from build123d import *

# Parameters (mm, degrees)
SKETCH1_R               = 30
SKETCH1_R_2             = 2
SKETCH1_R_3             = 6
BOSS_EXTRUDE1_DEPTH     = 12
SKETCH2_R               = 2.5
CUT_EXTRUDE1_DEPTH      = 31
CUT_EXTRUDE1_DEPTH_BACK = 31
SKETCH3_R               = 5
CUT_EXTRUDE2_DEPTH      = 5


with BuildPart() as part:
    # Sketch1 → Boss-Extrude1 (new body)
    with BuildSketch(Plane(origin=(0, 0, 0), x_dir=(1, 0, 0), z_dir=(0, 1, 0))):
        Circle(SKETCH1_R)
        with Locations((20, 0)):
            Circle(SKETCH1_R_2, mode=Mode.SUBTRACT)
        with Locations((10, -17.320508076)):
            Circle(SKETCH1_R_2, mode=Mode.SUBTRACT)
        with Locations((-10, -17.320508076)):
            Circle(SKETCH1_R_2, mode=Mode.SUBTRACT)
        with Locations((-20, 0)):
            Circle(SKETCH1_R_2, mode=Mode.SUBTRACT)
        with Locations((-10, 17.320508076)):
            Circle(SKETCH1_R_2, mode=Mode.SUBTRACT)
        with Locations((10, 17.320508076)):
            Circle(SKETCH1_R_2, mode=Mode.SUBTRACT)
        Circle(SKETCH1_R_3, mode=Mode.SUBTRACT)
    extrude(amount=BOSS_EXTRUDE1_DEPTH)

    # Sketch2 → Cut-Extrude1 (cut, two sides)
    with BuildSketch(Plane.XY) as cut_extrude1_sk:
        with Locations((0, 6)):
            Circle(SKETCH2_R)
    extrude(amount=CUT_EXTRUDE1_DEPTH, mode=Mode.SUBTRACT)
    extrude(cut_extrude1_sk.sketch, amount=-CUT_EXTRUDE1_DEPTH_BACK, mode=Mode.SUBTRACT)

    # Sketch3 → Cut-Extrude2 (cut)
    with BuildSketch(Plane(origin=(0, 12, 0), x_dir=(1, 0, 0), z_dir=(0, 1, 0))):
        with Locations((-10, 17.320508076)):
            Circle(SKETCH3_R)
        with Locations((10, 17.320508076)):
            Circle(SKETCH3_R)
        with Locations((20, 0)):
            Circle(SKETCH3_R)
        with Locations((10, -17.320508076)):
            Circle(SKETCH3_R)
        with Locations((-10, -17.320508076)):
            Circle(SKETCH3_R)
        with Locations((-20, 0)):
            Circle(SKETCH3_R)
    extrude(amount=-CUT_EXTRUDE2_DEPTH, mode=Mode.SUBTRACT)


solid = part.part
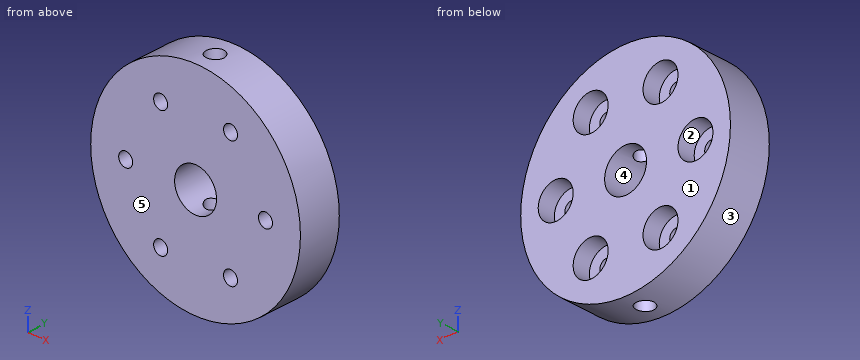
Could you check a few things on this model? Use its own coordinates, in mm. Face numbers are marked on the shaded views. A direction names the side the tool comes from. Coordinates: 2 decimals unless noted, no trailing zeros. Order: outer loops, then holes, each group sorted by start corner. A loop starts at its lowest first (then second) coordinate and runs counter-clockwise, first axis right, second up.
Q1. Which directions (+Z, -Z, +X, -X, +Y, -Y) give clear straight access to the entire face, cutting with the end or side of a thin tool? Please do the marked faces 1 and 2.
Q2. Will these pins go through, and if not, where does the flat tip stop? pin 1 (6 mm diameter, centred on y = 4.5, z = 23.5, fed in from +X); pin 2 (1 mm diameter, centred on x = 10, y = 4, fed in from -Z); pin 3 (8 mm diameter, centred on x = -10, z = -17.32, fed in from +Y).
Q3. Please list where these lines run through material, in increasing order: L1, parallel to X at y = 10.95, z = 0; L2, parallel to Z at x = 10, y = 4.5; L3, parallel to X at y = 4.5, z = -19.
Q4. Thinking about a two-plate mould opening in Z: for the marked faces 3, 4 and 5, which applies, released by +Z, released by -Z, zero draft, split by the parting line, or undercut?
Q5. Suppose I cut it at C-C on x = 0. Please give me the cut outline in (y, z), and give its area (3 significant figures).
Q6. Suppose I cut it at D-D on y = 1.5. Please give me the cut outline in (x, z), and give its area (3 significant figures).
Q7. Suppose I cut it at A-A on y = 4.5. Please give me the cut outline in (x, z).
Q8. Suppose I cut it at B-B on z = 16.5. Please give me the cut outline in (x, y).
Answer:
1. face 1: +Z, -Z, +X, -X, +Y
1. face 2: +Y
2. pin 1: stops at x = 21.9
2. pin 2: stops at z = -28.46
2. pin 3: stops at y = 7
3. L1: x = -30 to -25, -15 to -6, 6 to 15, 25 to 30
3. L2: z = -28.28 to -19.32, -15.32 to 15.32, 19.32 to 28.28
3. L3: x = -23.22 to -11.09, -8.91 to -2, 2 to 8.91, 11.09 to 23.22
4. face 3: split by the parting line
4. face 4: undercut
4. face 5: zero draft
5. outline: (0, -30) - (3.5, -30) - (3.5, -6) - (0, -6) - close; (0, 6) - (3.5, 6) - (3.5, 30) - (0, 30) - close; (8.5, -30) - (12, -30) - (12, -6) - (8.5, -6) - close; (8.5, 6) - (12, 6) - (12, 30) - (8.5, 30) - close
5. area: 336 mm2
6. outline: circle Ø60 at (0, 0); hole circle Ø4 at (-20, 0); hole circle Ø4 at (-10, -17.32); hole circle Ø4 at (-10, 17.32); hole circle Ø12 at (0, 0); hole circle Ø4 at (10, -17.32); hole circle Ø4 at (10, 17.32); hole circle Ø4 at (20, 0)
6. area: 2,640 mm2
7. outline: (-2, -29.93) - (-2, -5.66) arc R6 cw to (-2, 5.66) - (-2, 29.93) arc R30 ccw to start; (2, -29.93) arc R30 ccw to (2, 29.93) - (2, 5.66) arc R6 cw to (2, -5.66) - close; hole circle Ø4 at (-20, 0); hole circle Ø4 at (-10, -17.32); hole circle Ø4 at (-10, 17.32); hole circle Ø4 at (10, -17.32); hole circle Ø4 at (10, 17.32); hole circle Ø4 at (20, 0)
8. outline: (-25.05, 0) - (-11.82, 0) - (-11.82, 7) - (-14.93, 7) - (-14.93, 12) - (-25.05, 12) - close; (-8.18, 0) - (8.18, 0) - (8.18, 7) - (5.07, 7) - (5.07, 12) - (-5.07, 12) - (-5.07, 7) - (-8.18, 7) - close; (11.82, 0) - (25.05, 0) - (25.05, 12) - (14.93, 12) - (14.93, 7) - (11.82, 7) - close; hole circle Ø5 at (0, 6)
